For this review, use the dimensioned drawing (mm, ordinates from the lowest corner) and the shaded views. A direction names the side the tool comes from. Give positions to 0.01 mm unless a question says otherwise; leave off trailing zeros. Loops run counter-clockwise (first coordinate to the right, second up) from the corner with the lowest first, then second, coordinate; pieces in that order, holes last. Notation, with made-up numbers: M 5.5,86 L 34.5,86 A9 ccw 34.5,103 Z; hole C 62,-14 d4. An arc over 180 degrees is marked long. Use CSV: the item, a comma, the result in double quotes.
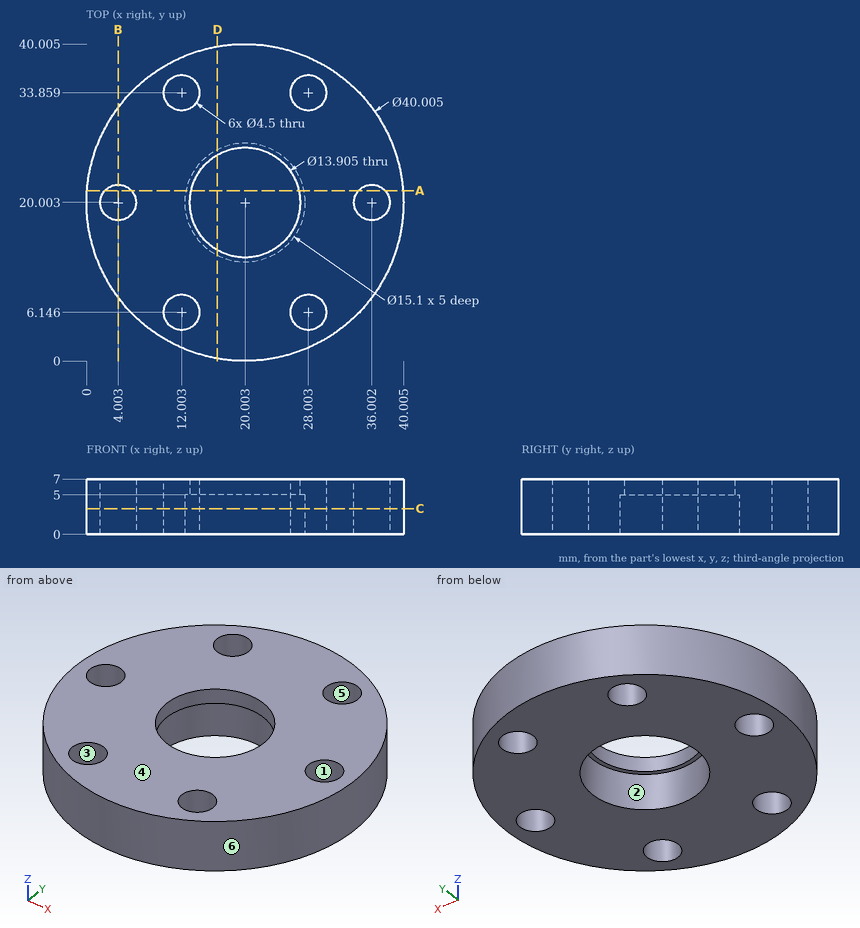
(1) The part is to be moulded in two halves that separate along X. For the marked faces 3, 4, 5 and 6, say which applies: released by +X, released by -X, zero draft, split by the parting line, or undercut.
A:
face 3,"undercut"
face 4,"zero draft"
face 5,"undercut"
face 6,"split by the parting line"
(2) We need section D-D on x = 16.5. State the section outline as (y, z) points (1 decimal), then the cut area to 3 significant figures.
A:
outline,"M 0.3,0 L 13.3,0 L 13.3,5 L 14,5 L 14,7 L 0.3,7 Z; M 26,5 L 26.7,5 L 26.7,0 L 39.7,0 L 39.7,7 L 26,7 Z"
area,"185 mm²"
(3) Wall thickness on line 1 along Y through (x, z) = (10, 2.5) (1 decimal); line 2 along X through (y, z) = (6.5, 5) (1 decimal); line 3 along Y through (x, z) = (13, 5.5) (1 decimal): over which ranges is each line inside the solid? List them lowest first. Write a range as [from, to].
A:
line 1,"[2.7, 5.1], [7.2, 32.8], [34.9, 37.3]"
line 2,"[5.2, 9.8], [14.2, 25.8], [30.2, 34.8]"
line 3,"[1.3, 4.1], [8.2, 31.8], [35.9, 38.7]"
(4) Machinability: for the marked faces 1 and 2, which of the approach directions +Z, -Z, +X, -X, +Y, -Y give a long, thin tool a straight path to every point of the face, cutting with its end or side? Answer none if there is none.
A:
face 1,"+Z, -Z"
face 2,"-Z"
(5) We need section C-C on z = 3.25. Count the separate pieces of the cut face and the enclosed holes in it.
A:
separate pieces,"1"
enclosed holes,"7"
(6) Clearance check with flat-ended pins moving along their axes: P1, Ø1.5, axis at x = 29, z = 5, coming from the -Y side; P2, Ø3, axis at y = 7.5, z = 3.5, coming from the -X side. State where each tip first meets the part, or that it passes through.
A:
P1,"y = 1.78"
P2,"x = 3.3"
(7) We need section B-B on x = 4. State the section outline as (y, z) points.
A:
outline,"M 8,0 L 17.75,0 L 17.75,7 L 8,7 Z; M 22.25,0 L 32,0 L 32,7 L 22.25,7 Z"
(8) We need section A-A on y = 21.5. State the section outline as (x, z) points, then the cut area to 3 significant figures.
A:
outline,"M 0.06,0 L 2.32,0 L 2.32,7 L 0.06,7 Z; M 5.68,0 L 12.6,0 L 12.6,5 L 13.21,5 L 13.21,7 L 5.68,7 Z; M 26.79,5 L 27.4,5 L 27.4,0 L 34.32,0 L 34.32,7 L 26.79,7 Z; M 37.68,0 L 39.95,0 L 39.95,7 L 37.68,7 Z"
area,"131 mm²"
